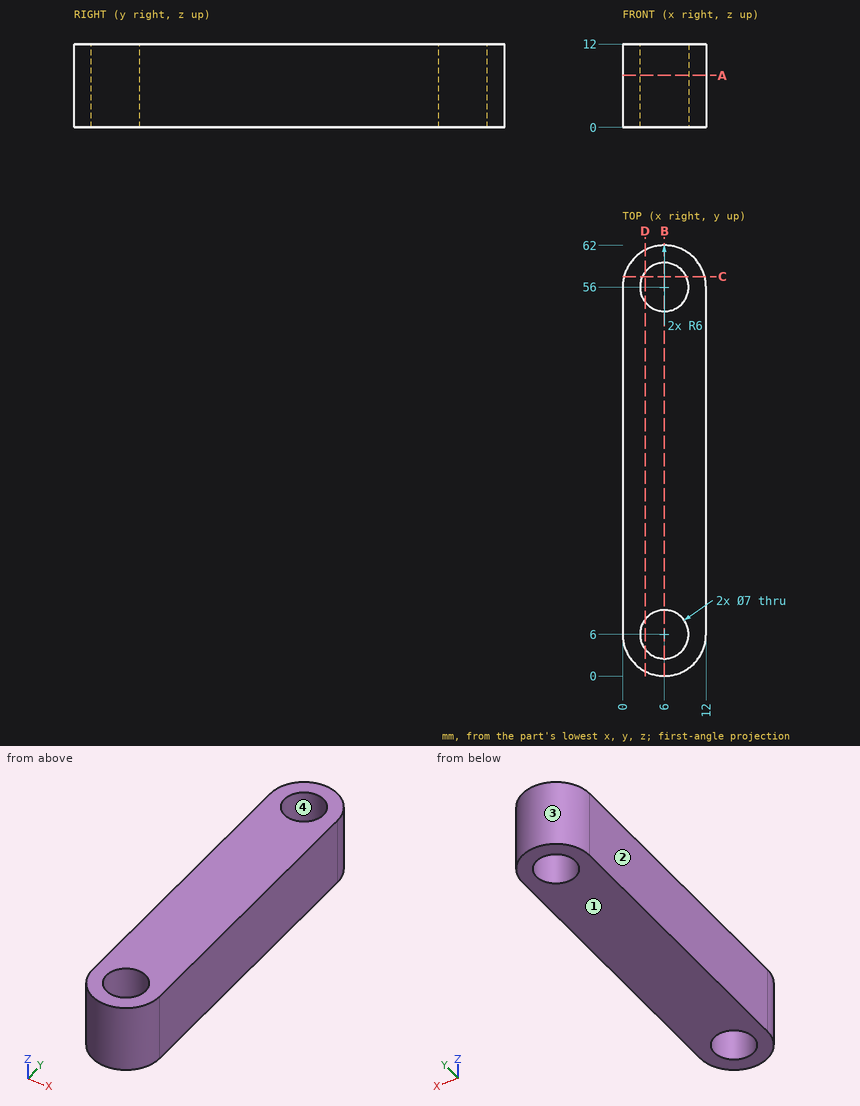
Can you work these out from the drawing? Everything is in mm from the part's minimum corner. Coordinates: 2 decimals unless noted, no trailing zeros. Write each loop counter-clockwise with the first axis right and the second up, starting at its lowest first coordinate (ties: lowest second). Pieces come first, ordered by that corner, then holes. Notation, with made-up numbers: (69.25, -3) -> (74.25, -3) arc R15 cw to (74.25, 21) -> close; hole circle Ø6 at (0, -40). An arc over 180 degrees is marked (long way). Write each question's results on one line, items separated by ' | '. Start each with the question number.
Item 1: I'm going to push flat-ended pins straight in: P1, Ø6.5, axis at x = 6, y = 6, coming from the +Z side (1 decimal); P2, Ø1.5, axis at y = 39, z = 7, coming from the -X side; P3, Ø6, axis at x = 9.5, z = 8, coming from the -Y side. Where does each tip first touch, or does it pass through?
Item 2: If we section it at D-D, the plane x = 3.25: Write out the boundary of the cut face in (y, z), and give its area (3 significant figures).
Item 3: Thinking about a two-plate mould opening in X: for the marked faces 1, 2, 3 and 4, which applies, released by +X, released by -X, zero draft, split by the parting line, or undercut?
Item 4: If we section it at B-B, the plane x = 6: Write out the boundary of the cut face in (y, z).
Item 5: If we section it at A-A, the plane z = 7.5: Write out the boundary of the cut face in (x, y), and give its area (3 significant figures).
Item 6: If we section it at C-C, the plane y = 57.5: Write out the boundary of the cut face in (x, z), and give its area (3 significant figures).
Item 7: Please list where these lines run through material, in increasing order: probe 1 along Y at (x, z) = (6, 5.75); probe 2 along Y at (x, z) = (8.75, 8.75); probe 3 along X at (y, z) = (59, 1).
Answer block:
1) P1: through | P2: x = 0 | P3: y = 0.02
2) outline: (0.67, 0) -> (3.83, 0) -> (3.83, 12) -> (0.67, 12) -> close; (8.17, 0) -> (53.83, 0) -> (53.83, 12) -> (8.17, 12) -> close; (58.17, 0) -> (61.33, 0) -> (61.33, 12) -> (58.17, 12) -> close | area: 624 mm²
3) face 1: zero draft | face 2: released by -X | face 3: split by the parting line | face 4: undercut
4) outline: (0, 0) -> (2.5, 0) -> (2.5, 12) -> (0, 12) -> close; (9.5, 0) -> (52.5, 0) -> (52.5, 12) -> (9.5, 12) -> close; (59.5, 0) -> (62, 0) -> (62, 12) -> (59.5, 12) -> close
5) outline: (0, 6) arc R6 ccw to (12, 6) -> (12, 56) arc R6 ccw to (0, 56) -> close; hole circle Ø7 at (6, 6); hole circle Ø7 at (6, 56) | area: 636 mm²
6) outline: (0.19, 0) -> (2.84, 0) -> (2.84, 12) -> (0.19, 12) -> close; (9.16, 0) -> (11.81, 0) -> (11.81, 12) -> (9.16, 12) -> close | area: 63.5 mm²
7) probe 1: 0 to 2.5, 9.5 to 52.5, 59.5 to 62 | probe 2: 0.67 to 3.83, 8.17 to 53.83, 58.17 to 61.33 | probe 3: 0.8 to 4.2, 7.8 to 11.2
